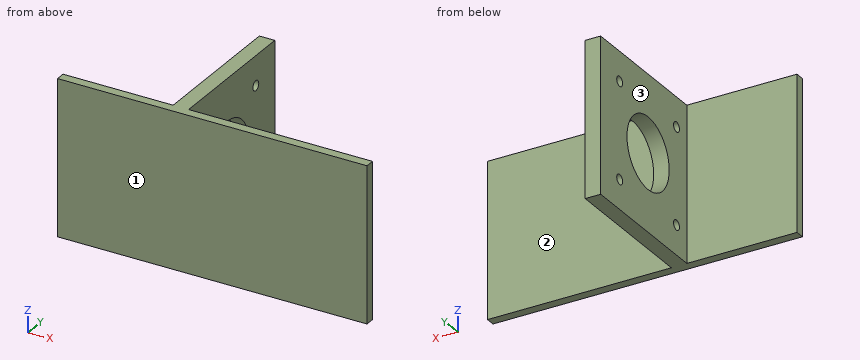
from build123d import *

# Parameters (mm, degrees)
SKETCH1_W           = 100
SKETCH1_H           = 50
BOSS_EXTRUDE1_DEPTH = 3
SKETCH2_W           = 5
SKETCH2_H           = 50
BOSS_EXTRUDE3_DEPTH = 47
SKETCH8_R           = 11.5
CUT_EXTRUDE3_DEPTH  = 82.577573944
SKETCH9_R           = 1.6
CUT_EXTRUDE4_DEPTH  = 82.577573944


with BuildPart() as part:
    # Sketch1 → Boss-Extrude1 (new body)
    with BuildSketch(Plane(origin=(0, 0, 0), x_dir=(1, 0, 0), z_dir=(0, 1, 0))):
        Rectangle(SKETCH1_W, SKETCH1_H)
    extrude(amount=BOSS_EXTRUDE1_DEPTH)

    # Sketch2 → Boss-Extrude3 (add)
    with BuildSketch(Plane(origin=(0, 3, 0), x_dir=(1, 0, 0), z_dir=(0, 1, 0))):
        with Locations((-11.912966351, 0)):
            Rectangle(SKETCH2_W, SKETCH2_H)
    extrude(amount=BOSS_EXTRUDE3_DEPTH)

    # Sketch8 → Cut-Extrude3 (cut, through all)
    with BuildSketch(Plane(origin=(-9.412966351, 0, 0), x_dir=(0, 0, -1), z_dir=(1, 0, 0))):
        with Locations((1.43e-06, 24.15)):
            Circle(SKETCH8_R)
    extrude(amount=-CUT_EXTRUDE3_DEPTH, mode=Mode.SUBTRACT)

    # Sketch9 → Cut-Extrude4 (cut, through all)
    with BuildSketch(Plane(origin=(-9.412966351, 0, 0), x_dir=(0, 0, -1), z_dir=(1, 0, 0))):
        with Locations((-15.49999857, 8.65)):
            Circle(SKETCH9_R)
        with Locations((-15.49999857, 39.65)):
            Circle(SKETCH9_R)
        with Locations((15.49999857, 39.65)):
            Circle(SKETCH9_R)
        with Locations((15.49999857, 8.65)):
            Circle(SKETCH9_R)
    extrude(amount=-CUT_EXTRUDE4_DEPTH, mode=Mode.SUBTRACT)


solid = part.part
Source: CAD feature listing. Evaluate the final solid. Frame: model axes, mm. Face numbers are marked on the shaded views. A direction names the side the tool comes from. Round coordinates to 2 decimals unless told otherwise and drop trailing zeros. Loops run counter-clockwise (first coordinate to the right, second up) from the corner with the lowest first, then second, coordinate; pieces in that order, holes last. Notation, with made-up numbers: (55, 35) -> (102, 35) arc R17 ccw to (102, 65) -> close; hole circle Ø11 at (24, 83). An arc over 180 degrees is marked (long way). Answer as a JSON object with one key per item and string values. Group by question number.
Q1. Section query B-B (z = -1). Output: boundary loops of the cut face in (x, y).
Q2. Access query for the marked faces 1, 2 and 3. Directions: +Z, -Z, +X, -X, +Y, -Y. A direction counts if a zero-diameter tool reaches every point of the face in a straight line with its end or side. Return the directions, or none.
Q3. Section query A-A (y = 39.65). Output: boundary loops of the cut face in (x, z), plus the area to 3 significant figures.
Q4. Contact query for flat-ended pins moving along their axis: P1, Ø3, axis at y = 39.65, z = -15.5, coming from the -X side; P2, Ø10, axis at x = -18.5, y = 34.5, coming from the +Z side; P3, Ø4, axis at y = 8.65, z = -15.5, coming from the -X side; P4, Ø5, axis at y = 44.5, z = -5, coming from the +X side. Output: stop coordinate, or through.
Q5. Section query C-C (y = 24.15). Output: boundary loops of the cut face in (x, z).
Q6. Ray query, line 1 (X direction, y = 11, z = 3); line 2 (Y direction, x = -5, z = -16); line 3 (Z direction, x = -12, y = 33.5). Return the intervals inside material, ascending. Write a range as from..to.
Q7. Section query D-D (x = -36.5). Output: boundary loops of the cut face in (y, z), plus the area to 3 significant figures.
Completed:
{
 "1": {"outline": "(-50, 0) -> (50, 0) -> (50, 3) -> (-9.41, 3) -> (-9.41, 12.69) -> (-14.41, 12.69) -> (-14.41, 3) -> (-50, 3) -> close; (-14.41, 35.61) -> (-9.41, 35.61) -> (-9.41, 50) -> (-14.41, 50) -> close"},
 "2": {"face 1": "+Z, -Z, +X, -X, -Y", "face 2": "+Z, -Z, +X, +Y", "face 3": "+Z, -Z, -X, +Y"},
 "3": {"outline": "(-14.41, -25) -> (-9.41, -25) -> (-9.41, -17.1) -> (-14.41, -17.1) -> close; (-14.41, -13.9) -> (-9.41, -13.9) -> (-9.41, 13.9) -> (-14.41, 13.9) -> close; (-14.41, 17.1) -> (-9.41, 17.1) -> (-9.41, 25) -> (-14.41, 25) -> close", "area": "218 mm²"},
 "4": {"P1": "through", "P2": "z = 25", "P3": "x = -14.41", "P4": "x = -9.41"},
 "5": {"outline": "(-14.41, -25) -> (-9.41, -25) -> (-9.41, -11.5) -> (-14.41, -11.5) -> close; (-14.41, 11.5) -> (-9.41, 11.5) -> (-9.41, 25) -> (-14.41, 25) -> close"},
 "6": {"line 1": "-14.41..-9.41", "line 2": "0..3", "line 3": "-25..-6.7, 6.7..25"},
 "7": {"outline": "(0, -25) -> (3, -25) -> (3, 25) -> (0, 25) -> close", "area": "150 mm²"}
}
